Can you work these out from the model? Positions are in its coordinate system, mm. Face numbers are marked on the shaded views. A direction names the side the tool comes from. Give positions to 0.01 mm unless a question says otherwise; leave off trailing zeros. Loops run counter-clockwise (first coordinate to the right, second up) from the corner with the lowest first, then second, coordinate; pieces in that order, holes last. Notation, with made-up numbers: M -24,74 L 27,74 A15 ccw 27,99 Z; hole C 4.5,22.5 d4. An arc over 180 degrees is marked long. Use CSV: the item, a comma, the result in double quotes.
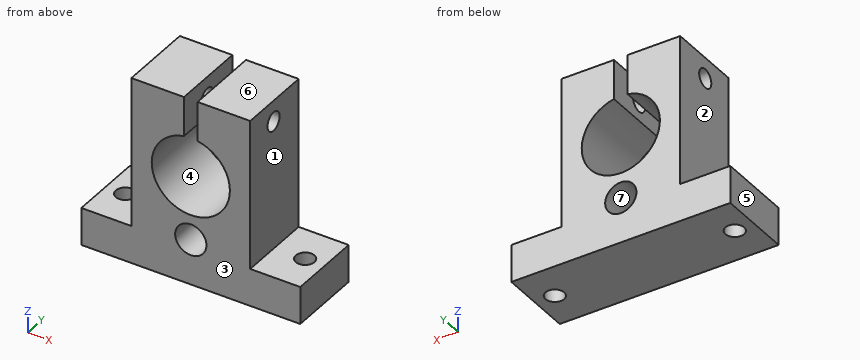
from build123d import *

# Parameters (mm, degrees)
F0_R     = 5
F1_DEPTH = 24
F3_D     = 6
F5_D     = 6


with BuildPart() as f1:
    # F0 (on Front) → F1 (new body)
    with BuildSketch(Plane.XZ):
        with BuildLine():
            Line((18.38709, 38.646828), (1.561872, 38.646828))
            Line((1.561872, 38.646828), (1.561872, -9.353172))
            Line((1.561872, -9.353172), (-14.438128, -9.353172))
            Line((-14.438128, -9.353172), (-14.438128, -21.353172))
            Line((-14.438128, -21.353172), (1.561872, -21.353172))
            Line((1.561872, -21.353172), (39.561872, -21.353172))
            Line((39.561872, -21.353172), (55.561872, -21.353172))
            Line((55.561872, -21.353172), (55.561872, -9.353172))
            Line((55.561872, -9.353172), (39.561872, -9.353172))
            Line((39.561872, -9.353172), (39.561872, 38.646828))
            Line((39.561872, 38.646828), (22.736653, 38.646828))
            Line((22.736653, 38.646828), (22.736653, 25.956187))
            ThreePointArc((22.736653, 25.956187), (20.561872, 1.146828), (18.38709, 25.956187))
            Line((18.38709, 25.956187), (18.38709, 38.646828))
        make_face()
        with Locations((20.561872, -6.853172)):
            Circle(F0_R, mode=Mode.SUBTRACT)
    extrude(amount=F1_DEPTH)

    # F3 (through all)
    with Locations(Plane.YZ.offset(39.561872)):
        with Locations((-12.408947, 31.925292)):
            Hole(F3_D / 2)

    # F5 (through all)
    with Locations(Plane.XY.offset(-9.353172)):
        with Locations((-8.209684, -11.887997), (49.306241, -11.887997)):
            Hole(F5_D / 2)


solid = f1.part
Q1. If we mould it in two halves opening along X, with no side actions, what happens to the marked faces 4, 5, 6 and 7? For each: released by +X, released by -X, zero draft, split by the parting line, or undercut.
Model answer:
face 4,"undercut"
face 5,"released by -X"
face 6,"zero draft"
face 7,"undercut"
Q2. I'm going to push flat-ended pins straight in: P1, Ø8, axis at x = 51, y = -13.5, coming from the +Z side; P2, Ø1, axis at y = -11.5, z = 9.5, coming from the -X side; P3, Ø6.5, axis at y = -18, z = 34.5, coming from the +X side. Where does each tip first touch, or does it pass through?
Model answer:
P1,"z = -9.35"
P2,"x = 1.56"
P3,"x = 39.56"
Q3. I want a section at A-A, the plane y = -13.5. State how many separate pieces and enclosed holes the cut face has, then the cut area to 3 significant figures.
Model answer:
separate pieces,"5"
enclosed holes,"1"
area,"1,730 mm2"
Q4. I want a section at D-D, the plane x = 10. Please give me the cut outline in (y, z).
Model answer:
outline,"M -24,-21.35 L 0,-21.35 L 0,6.96 L -24,6.96 Z; M -24,20.33 L 0,20.33 L 0,38.65 L -24,38.65 Z; hole C -12.41,31.93 d6"
Q5. I want a section at C-C, the plane x = -6. Please give me the cut outline in (y, z).
Model answer:
outline,"M -24,-21.35 L -13.92,-21.35 L -13.92,-9.35 L -24,-9.35 Z; M -9.86,-21.35 L 0,-21.35 L 0,-9.35 L -9.86,-9.35 Z"
Q6. For the marked faces 1, 2 and 3, which set-ups out of +Z, -Z, +X, -X, +Y, -Y let a thin tool reach every point of the face, with its end or its side?
Model answer:
face 1,"+Z, +X, +Y, -Y"
face 2,"+Z, -X, +Y, -Y"
face 3,"+Z, -Z, +X, -X, -Y"
Q7. Please list where these lines run through material, in increasing order: L1, parallel to X at y = -15.25, z = 28; L2, parallel to Z at x = 37, y = -12.5; L3, parallel to Z at x = 25, y = -17. Write a range as from..to.
Model answer:
L1,"1.56..18.39, 22.74..39.56"
L2,"-21.35..28.93, 34.92..38.65"
L3,"-21.35..-9.16, -4.55..1.96, 25.33..38.65"
Q8. I want a section at B-B, the plane z = -3.5. Please give me the cut outline in (x, y), then the cut area to 3 significant figures.
Model answer:
outline,"M 1.56,-24 L 16.85,-24 L 16.85,0 L 1.56,0 Z; M 24.27,-24 L 39.56,-24 L 39.56,0 L 24.27,0 Z"
area,"734 mm2"
